```python
from build123d import *

# Parameters (mm, degrees)
SKETCH1_R               = 3.5
SKETCH1_R_2             = 16
BOSS_EXTRUDE2_DEPTH     = 60
CUT_EXTRUDE6_DEPTH      = 1
CUT_EXTRUDE6_DEPTH_BACK = 2
SKETCH7_R               = 2
CUT_EXTRUDE7_DEPTH      = 59
SKETCH8_R               = 18
SKETCH8_R_2             = 16
BOSS_EXTRUDE3_DEPTH     = 2
CUT_EXTRUDE8_START      = 6
SKETCH9_R               = 24
CUT_EXTRUDE8_DEPTH      = 3
LPATTERN1_COUNT         = 9
LPATTERN1_PITCH         = 6


with BuildPart() as part:
    # Sketch1 → Boss-Extrude2 (new body)
    with BuildSketch(Plane(origin=(0, 0, 0), x_dir=(1, 0, 0), z_dir=(0, 1, 0))):
        with BuildLine():
            Line((-21, -22.5), (21, -22.5))
            ThreePointArc((21, -22.5), (23.828427125, -21.328427125), (25, -18.5))
            Line((25, -18.5), (25, 18.5))
            ThreePointArc((25, 18.5), (23.828427125, 21.328427125), (21, 22.5))
            Line((21, 22.5), (-21, 22.5))
            ThreePointArc((-21, 22.5), (-23.828427125, 21.328427125), (-25, 18.5))
            Line((-25, 18.5), (-25, -18.5))
            ThreePointArc((-25, -18.5), (-23.828427125, -21.328427125), (-21, -22.5))
        make_face()
        with Locations((18.688018935, 16.819217042)):
            Circle(SKETCH1_R, mode=Mode.SUBTRACT)
        with Locations((19.819217042, -15.688018935)):
            Circle(SKETCH1_R, mode=Mode.SUBTRACT)
        with Locations((-12.688018935, -16.819217042)):
            Circle(SKETCH1_R, mode=Mode.SUBTRACT)
        with Locations((-13.819217042, 15.688018935)):
            Circle(SKETCH1_R, mode=Mode.SUBTRACT)
        with Locations((3, 0)):
            Circle(SKETCH1_R_2, mode=Mode.SUBTRACT)
    extrude(amount=BOSS_EXTRUDE2_DEPTH)

    # Sketch6 → Cut-Extrude6 (cut, two sides)
    with BuildSketch(Plane(origin=(0, 60, 0), x_dir=(1, 0, 0), z_dir=(0, 1, 0))) as cut_extrude6_sk:
        with BuildLine():
            Line((-13, 2), (-21, 2))
            ThreePointArc((-21, 2), (-23, 0), (-21, -2))
            Line((-21, -2), (-13, -2))
            ThreePointArc((-13, -2), (-12.93746943, -1.999022243), (-12.875, -1.996089928))
            ThreePointArc((-12.875, -1.996089928), (-13, 0), (-12.875, 1.996089928))
            ThreePointArc((-12.875, 1.996089928), (-12.93746943, 1.999022243), (-13, 2))
        make_face()
    extrude(amount=CUT_EXTRUDE6_DEPTH, mode=Mode.SUBTRACT)
    extrude(cut_extrude6_sk.sketch, amount=-CUT_EXTRUDE6_DEPTH_BACK, mode=Mode.SUBTRACT)

    # Sketch7 → Cut-Extrude7 (cut, through all)
    with BuildSketch(Plane(origin=(0, 58, 0), x_dir=(1, 0, 0), z_dir=(0, 1, 0))):
        with Locations((-21, 0)):
            Circle(SKETCH7_R)
    extrude(amount=-CUT_EXTRUDE7_DEPTH, mode=Mode.SUBTRACT)

    # Sketch8 → Boss-Extrude3 (add)
    with BuildSketch(Plane.XZ):
        with Locations((3, 0)):
            Circle(SKETCH8_R)
        with Locations((3, 0)):
            Circle(SKETCH8_R_2, mode=Mode.SUBTRACT)
    extrude(amount=BOSS_EXTRUDE3_DEPTH)

    # Sketch9 → Cut-Extrude8 (cut)
    with BuildSketch(Plane(origin=(0, 0, 0), x_dir=(1, 0, 0), z_dir=(0, 1, 0)).offset(CUT_EXTRUDE8_START)):
        with Locations((45, 0)):
            Circle(SKETCH9_R)
        with Locations((0, 42.5)):
            Circle(SKETCH9_R)
        with Locations((0, -42.5)):
            Circle(SKETCH9_R)
    cut_extrude8 = extrude(amount=CUT_EXTRUDE8_DEPTH, mode=Mode.SUBTRACT)

    # LPattern1: Cut-Extrude8 ×9
    with Locations(*[(0, i * LPATTERN1_PITCH, 0) for i in range(1, LPATTERN1_COUNT)]):
        add(cut_extrude8, mode=Mode.SUBTRACT)


solid = part.part
```
The listing builds one solid part. Answer for the finished solid, in the listing's coordinates (mm). A direction names the side the tool comes from. Coordinates: 2 decimals unless noted, no trailing zeros. Write each loop counter-clockwise with the first axis right and the second up, starting at its lowest first coordinate (ties: lowest second). Pieces come first, ordered by that corner, then holes. Notation, with made-up numbers: M 33,-14 L 41,-14 A21 ccw 41,22 Z; hole C 75.25,-2.5 d8. An arc over 180 degrees is marked long. Use a Markdown table: item, result. Add a question column.
1. For a pull along X with two mould halves and no side action, classify faces 1 (the flat face through (0, 6, -21)), 2 (the flat face through (23, 12, 0)), 3 (the flat face through (0, 9, -21)), 4 (the cylindrical face through (21, 37, 0)) as +X half, -X half, draft (parallel to the pull), parting line (faces both ways), or undercut.
2. Given P1, Ø10, axis at x = -2, z = -5, coming from the -Y side; P2, Ø4.5, axis at x = 4.5, z = -21, coming from the -Y side; P3, Ø1.2, axis at x = -16.5, z = 0.5, coming from the +Y side; P4, Ø1.5, axis at y = 13, z = -1, coming from the +X side, each flat-ended and moving along its own axis, determine where each tip first touches the part or whether it passes through.
3. Straight lines are drawn through the part: line 1 along X through (y, z) = (35, 0); line 2 along X through (y, z) = (27.5, 1.5); line 3 along Z through (x, y) = (20, 48.5). For each, find the intervals that lie inside material, in ascending order. Write a range as [from, to].
4. Which of the six approach directions +Z, -Z, +X, -X, +Y, -Y give full straight-line access (tool end or side, diameter ignored) to faces 5 (the flat face through (0, 21, 21)), 6 (the flat face through (-17, 59, 2)), 7 (the flat face through (23, 45, 0))?
5. Section A-A (y = 16) is taken. Give the vertices of the cut face in (x, z), plus the area to 3 significant figures.
6. Section B-B (z = 0) is taken. Count the separate pieces of the cut face and the enclosed holes in it, plus the area to 3 significant figures.
7. Section C-C (y = 8) is taken. Give the vertices of the cut face in (x, z), plus the area to 3 significant figures.
Data:
| question | item | result |
|---|---|---|
| 1 | face 1 | undercut |
| 1 | face 2 | draft |
| 1 | face 3 | undercut |
| 1 | face 4 | +X half |
| 2 | P1 | passes through |
| 2 | P2 | stops at y = 0 |
| 2 | P3 | stops at y = 58 |
| 2 | P4 | stops at x = 21.06 |
| 3 | line 1 | x = [-25, -23], [-19, -13], [19, 25] |
| 3 | line 2 | x = [-25, -22.32], [-19.68, -12.93], [18.93, 25] |
| 3 | line 3 | z = [-22.5, -20.06], [-13.57, 12.19], [19.18, 22.5] |
| 4 | face 5 | +Z |
| 4 | face 6 | +Y |
| 4 | face 7 | +X |
| 5 | outline | M -25,-18.5 A4 ccw -21,-22.5 L 21,-22.5 A4 ccw 25,-18.5 L 25,18.5 A4 ccw 21,22.5 L -21,22.5 A4 ccw -25,18.5 Z; hole C -21,0 d4; hole C -13.82,-15.69 d7; hole C -12.69,16.82 d7; hole C 3,0 d32; hole C 18.69,-16.82 d7; hole C 19.82,15.69 d7 |
| 5 | area | 1,270 mm2 |
| 6 | separate pieces | 3 |
| 6 | enclosed holes | 0 |
| 6 | area | 728 mm2 |
| 7 | outline | M -25,-18.5 A4 ccw -21,-22.5 L -13.27,-22.5 A24 cw 13.27,-22.5 L 21,-22.5 A4 ccw 25,-18.5 L 25,-13.27 A24 cw 25,13.27 L 25,18.5 A4 ccw 21,22.5 L 13.27,22.5 A24 cw -13.27,22.5 L -21,22.5 A4 ccw -25,18.5 Z; hole C -21,0 d4; hole C -13.82,-15.69 d7; hole C -12.69,16.82 d7; hole C 3,0 d32; hole C 18.69,-16.82 d7; hole C 19.82,15.69 d7 |
| 7 | area | 1,050 mm2 |
